Autodesk Inventor part; units mm, degrees
ref_plane "Start plane" through (0, 0, 0) normal (0, 0, 1) x (1, 0, 0)
ref_plane "End plane" through (0, 0, 50) normal (0, 0, 1) x (1, 0, 0)
ref_plane "YZ Plane" through (0, 0, 0) normal (1, 0, 0) x (0, 1, 0)
ref_plane "Start plane" through (0, 0, 0) normal (0, 0, 1) x (1, 0, 0)
ref_plane "End plane" through (0, 0, 50) normal (0, 0, 1) x (1, 0, 0)
sketch "Sketch" plane through (0, 0, 0) normal (0, 0, 1) x (1, 0, 0)
  circle A0 centre (0, 0) radius 45
  dimension "d0" = 90
extrude "Body" add sketch "Sketch" along normal blind 90
sketch "Sketch5" plane through (0, 0, 0) normal (0, 0, -1) x (-1, 0, 0)
  line L0 (-37.5, -37.5) -> (-37.5, 42.1268)
  point P0 (0, 0)
ref_plane "Work Plane4" through (37.5, -24.8747, 0) normal (0.8333333, -0.5527708, 0) x (0.5527708, 0.8333333, 0)
sketch "Sketch6" plane through (37.5, -24.8747, 0) normal (0.8333333, -0.5527708, 0) x (0.5527708, 0.8333333, 0)
  line L0 (-45, 0) -> (45, 0)
  line L1 (-45, 0) -> (-45, 90)
  line L2 (-45, 0) -> (66.6399, 52.0585)
  line L3 (-45, 0) -> (55.6312, 0) construction
  line L4 (66.6399, 52.0585) -> (66.6399, 0)
  line L5 (-45, 0) -> (66.6399, 0)
  point P0 (0, 0)
  point P1 (45, 90)
  dimension "d9" = 25
extrude "Extrusion2" cut sketch "Sketch6" against normal blind 124.75
sketch "Sketch9" plane through (0, 0, 20.9838) normal (0.233611, 0.3521819, -0.9063078) x (-0.8333333, 0.5527708, 0)
  line L0 (0, -12.6785) -> (0, 0.5509) construction
  line L1 (0, -12.6785) -> (11.8004, -12.6785) construction
  ellipse E0 centre (0, 0) end of major axis (0, -49.652) minor radius 45
  line L2 (0, 49.652) -> (100.5638, 49.652) construction
  ellipse E1 centre (0, 29.1675) end of major axis (45, 29.1675) minor radius 40.7839
  line L3 (0, 69.9513) -> (0, -11.6164)
  point P0 (0, -8.8682)
sketch "Sketch7" plane through (0, 0, 90) normal (0, 0, 1) x (1, 0, 0)
  line L0 (0, 0) -> (37.25, 0) construction
  line L1 (144.8898, -42.1091) -> (-141.4436, 147.8231)
  circle A0 centre (0, 0) radius 45
  line L2 (17.2325, 42.5693) -> (30.6003, 33.7021)
  circle A1 centre (0, 0) radius 45
  line L3 (24.8747, 37.5) -> (0, 0)
  point P0 (20.5907, 31.0417)
  point P1 (20.5907, 31.0417)
  point P2 (-31.0417, 20.5907)
  point P3 (-31.0417, 20.5907)
  point P4 (-20.5907, -31.0417)
  point P5 (-20.5907, -31.0417)
  point P6 (31.0417, -20.5907)
  point P7 (31.0417, -20.5907)
  point P8 (25.3722, 36.5516)
  dimension "d12" = 37.25
  dimension "d26" = 360
hole "Hole1" at (20.5907, 31.0417, 90) at (-31.0417, 20.5907, 90) at (-20.5907, -31.0417, 90) at (31.0417, -20.5907, 90) direction (0, 0, -1) diameter 8 end up to surface
sketch "Sketch10" plane through (0, 0, 90) normal (0, 0, 1) x (1, 0, 0)
  point P0 (0, 0)
equation "\"G_H\" = 75"
equation "\"G_L\" = d8"
equation "\"G_OFFSET_START\" = 0"
equation "\"G_OFFSET_END\" = 0"
equation "\"G_D\" = 75"
properties part number "PN EN 10060 - 75 - 50" material "Steel, Mild"
For this review, take the finished solid that the model builds, in its own axes (mm). Round coordinates to 2 decimals unless told otherwise and drop trailing zeros. Write each loop counter-clockwise with the first axis right and the second up, starting at its lowest first coordinate (ties: lowest second). Pieces come first, ordered by that corner, then holes. Notation, with made-up numbers: (83.25, 22) -> (132.25, 22) arc R34 ccw to (132.25, 53) -> close; hole circle Ø10 at (-4.75, 69). An arc over 180 degrees is marked (long way). Use CSV: the item, a comma, the result in double quotes.
(1) Draft analysis for pull direction X (two halves, no side actions). For faces 1 (the face through (-1, 1, 90)), 2 (the face through (-32.243, 16.775, 54.05)), 3 (the face through (0.18, -0.87, 20.69)), state which applies: +X half, -X half, draft (parallel to the pull), parting line (faces both ways), or undercut.
Computed values:
face 1,"draft"
face 2,"undercut"
face 3,"+X half"
(2) Consider section B-B, the plane x = -15. Give the boundary of the cut face in (y, z).
Computed values:
outline,"(-42.43, 0.63) -> (42.43, 33.6) -> (42.43, 90) -> (-42.43, 90) -> close"
(3) Consider section C-C, the plane y = 0. Give the boundary of the cut face in (x, z).
Computed values:
outline,"(-45, 9.38) -> (45, 32.58) -> (45, 90) -> (-45, 90) -> close"
(4) To check wall thickness, follow L1, parallel to X at y = -21.5, z = 76.5; L2, parallel to Y at x = 23, z = 59; L3, parallel to X at y = 31, z = 48.5. State the ranges of each line that lie inside material, in increasing order. Write a range as [from, to].
Computed values:
L1,"[-39.53, 27.15], [34.94, 39.53]"
L2,"[-38.68, 27.85], [34.23, 38.68]"
L3,"[-32.62, 16.59], [24.59, 32.62]"
(5) Clearance check with flat-ended pins moving along their axes: P1, Ø10, axis at y = -12.5, z = 33, coming from the -X side; P2, Ø8, axis at x = -5, z = 50, coming from the -Y side; P3, Ø8, axis at x = 34.5, y = 35, coming from the +Z side; P4, Ø10, axis at x = 14, z = 61.5, coming from the -Y side. State where each tip first meets the part, or that it passes through.
Computed values:
P1,"x = -44.37"
P2,"y = -44.99"
P3,"through"
P4,"y = -44.09"
(6) Consider section A-A, the plane z = 46.5. Give the boundary of the cut face in (x, y), plus the area to 3 significant figures.
Computed values:
outline,"circle Ø90 at (0, 0); hole circle Ø8 at (-31.04, 20.59); hole circle Ø8 at (-20.59, -31.04); hole circle Ø8 at (20.59, 31.04); hole circle Ø8 at (31.04, -20.59)"
area,"6,160 mm²"
